The model under review builds one solid part; all positions refer to its coordinate system, in mm. A direction names the side the tool comes from. Give positions to 0.01 mm unless a question says otherwise; leave off trailing zeros. Order: outer loops, then holes, each group sorted by start corner. A loop starts at its lowest first (then second) coordinate and runs counter-clockwise, first axis right, second up. Notation, with made-up numbers: (-12.75, 49) - (21.25, 49) arc R27 ccw to (21.25, 87) - close; hole circle Ø7 at (66, 2). An arc over 180 degrees is marked (long way). Use CSV: the item, a comma, the result in double quotes.
Autodesk Inventor part; units mm, degrees
ref_plane "rail_to_adjusting_block_XY" through (0, 0, -37.5) normal (0, 1, 0) x (1, 0, 0)
ref_plane "rail_to_adjusting_block_YZ" through (0, 0, -37.5) normal (1, 0, 0) x (0, 0, -1)
ref_plane "rail_to_adjusting_block_ZX" through (0, 0, -37.5) normal (0, 0, -1) x (0, 1, 0)
sketch "Sketch_12" plane through (0, 0, 0) normal (0, 0, 1) x (1, 0, 0)
  line L0 (-2.5, 3.7) -> (-2.5, 3.1084)
  line L1 (-2.5, 3.1084) -> (-2.3242, 3.0098)
  arc A0 (-2.1007, 2.75) -> (-2.3242, 3.0098) centre (-2.5686, 2.5736) ccw
  line L2 (-2.1007, 2.75) -> (-1.5, 2.75)
  line L3 (-1.5, 2.75) -> (-1.5, 2.25)
  line L4 (-1.5, 2.25) -> (-2.1007, 2.25)
  arc A1 (-2.3242, 1.9902) -> (-2.1007, 2.25) centre (-2.5686, 2.4264) ccw
  line L5 (-2.3242, 1.9902) -> (-2.5, 1.8917)
  line L6 (-2.5, 1.8917) -> (-2.5, 0.3)
  line L7 (-2.5, 0.3) -> (-2.2, 0)
  line L8 (-2.2, 0) -> (2.2, 0)
  line L9 (2.2, 0) -> (2.5, 0.3)
  line L10 (2.5, 0.3) -> (2.5, 1.8917)
  line L11 (2.5, 1.8917) -> (2.3242, 1.9902)
  arc A2 (2.1007, 2.25) -> (2.3242, 1.9902) centre (2.5686, 2.4263) ccw
  line L12 (2.1007, 2.25) -> (1.5, 2.25)
  line L13 (1.5, 2.25) -> (1.5, 2.75)
  line L14 (1.5, 2.75) -> (2.1007, 2.75)
  arc A3 (2.3242, 3.0098) -> (2.1007, 2.75) centre (2.5686, 2.5737) ccw
  line L15 (2.3242, 3.0098) -> (2.5, 3.1084)
  line L16 (2.5, 3.1084) -> (2.5, 3.7)
  line L17 (2.5, 3.7) -> (2.2, 4)
  line L18 (2.2, 4) -> (-2.2, 4)
  line L19 (-2.2, 4) -> (-2.5, 3.7)
extrude "Extrusion1" add sketch "Sketch_12" along normal mid plane 85
sketch "Sketch2" plane through (-2.2, 4, 42.5) normal (0, 1, 0) x (1, 0, 0)
  point P0 (2.2, 80)
hole "Hole1" at (0, 4, -37.5) direction (0, -1, 0) diameter 2.4 depth 4 counterbore diameter 3.5 counterbore depth 1
pattern_linear "Rectangular Pattern1" count 6 spacing 15 along (0, 0, 1) of "Hole1"
ref_plane "rail_to_adjusting_block_XY" through (0, 0, -37.5) normal (0, 1, 0) x (1, 0, 0)
ref_plane "rail_to_adjusting_block_YZ" through (0, 0, -37.5) normal (1, 0, 0) x (0, 0, -1)
ref_plane "rail_to_adjusting_block_ZX" through (0, 0, -37.5) normal (0, 0, -1) x (0, 1, 0)
ref_plane "screw_1_XY" through (0, 3, 37.5) normal (0, -1, 0) x (1, 0, 0)
ref_plane "screw_1_YZ" through (0, 3, 37.5) normal (1, 0, 0) x (0, 0, 1)
ref_plane "screw_1_ZX" through (0, 3, 37.5) normal (0, 0, 1) x (0, -1, 0)
ref_plane "screw_2_XY" through (0, 3, 22.5) normal (0, -1, 0) x (1, 0, 0)
ref_plane "screw_2_YZ" through (0, 3, 22.5) normal (1, 0, 0) x (0, 0, 1)
ref_plane "screw_2_ZX" through (0, 3, 22.5) normal (0, 0, 1) x (0, -1, 0)
ref_plane "screw_3_XY" through (0, 3, 7.5) normal (0, -1, 0) x (1, 0, 0)
ref_plane "screw_3_YZ" through (0, 3, 7.5) normal (1, 0, 0) x (0, 0, 1)
ref_plane "screw_3_ZX" through (0, 3, 7.5) normal (0, 0, 1) x (0, -1, 0)
ref_plane "screw_4_XY" through (0, 3, -7.5) normal (0, -1, 0) x (1, 0, 0)
ref_plane "screw_4_YZ" through (0, 3, -7.5) normal (1, 0, 0) x (0, 0, 1)
ref_plane "screw_4_ZX" through (0, 3, -7.5) normal (0, 0, 1) x (0, -1, 0)
ref_plane "screw_5_XY" through (0, 3, -22.5) normal (0, -1, 0) x (1, 0, 0)
ref_plane "screw_5_YZ" through (0, 3, -22.5) normal (1, 0, 0) x (0, 0, 1)
ref_plane "screw_5_ZX" through (0, 3, -22.5) normal (0, 0, 1) x (0, -1, 0)
ref_plane "screw_6_XY" through (0, 3, -37.5) normal (0, -1, 0) x (1, 0, 0)
ref_plane "screw_6_YZ" through (0, 3, -37.5) normal (1, 0, 0) x (0, 0, 1)
ref_plane "screw_6_ZX" through (0, 3, -37.5) normal (0, 0, 1) x (0, -1, 0)
ref_plane "to_block_XY" through (0, 4, 21.25) normal (0, 0, 1) x (1, 0, 0)
ref_plane "to_block_YZ" through (0, 4, 21.25) normal (1, 0, 0) x (0, 1, 0)
ref_plane "to_block_ZX" through (0, 4, 21.25) normal (0, 1, 0) x (0, 0, 1)
ref_plane "to_block_2_XY" through (0, 4, -21.25) normal (0, 0, 1) x (1, 0, 0)
ref_plane "to_block_2_YZ" through (0, 4, -21.25) normal (1, 0, 0) x (0, 1, 0)
ref_plane "to_block_2_ZX" through (0, 4, -21.25) normal (0, 1, 0) x (0, 0, 1)
ref_plane "to_kue_XY" through (0, 0, 0) normal (0, 1, 0) x (1, 0, 0)
ref_plane "to_kue_YZ" through (0, 0, 0) normal (1, 0, 0) x (0, 0, -1)
ref_plane "to_kue_ZX" through (0, 0, 0) normal (0, 0, -1) x (0, 1, 0)
properties part number "SSE2B6-85_r"
Item 1: Take a section at B-B, the plane y = 1. Give the boundary of the cut face in (x, z), and give its area (3 significant figures).
Results list:
outline,"(-2.5, -42.5) - (2.5, -42.5) - (2.5, 42.5) - (-2.5, 42.5) - close; hole circle Ø2.4 at (0, -37.5); hole circle Ø2.4 at (0, -22.5); hole circle Ø2.4 at (0, -7.5); hole circle Ø2.4 at (0, 7.5); hole circle Ø2.4 at (0, 22.5); hole circle Ø2.4 at (0, 37.5)"
area,"398 mm2"
Item 2: Clearance check with flat-ended pins moving along their axes: pin 1 (0.6 mm diameter, centred on y = 2.5, z = -2.5, fed in from +X); pin 2 (1.9 mm diameter, centred on x = 0, z = 22.5, fed in from +Y); pin 3 (3 mm diameter, centred on x = 0, z = -22.5, fed in from +Y). State where each tip first meets the part, or that it passes through.
Results list:
pin 1,"stops at x = 2.12"
pin 2,"passes through"
pin 3,"stops at y = 3"
Item 3: Mouldability with a two-part tool opening along Z and no side actions: class faces 3 (the face through (0, 2, -42.5)), 4 (the face through (0, 4, -1)), 5 (the face through (-0.08, 3.49, -24.25)) as pulls with the +Z half, pulls with the -Z half, needs draft (parallel to the pull), parting line crosses it, or undercut.
Results list:
face 3,"pulls with the -Z half"
face 4,"needs draft"
face 5,"undercut"
Item 4: Wall thickness on L1, parallel to Y at x = -1.8, z = -35.5; L2, parallel to X at y = 1.05, z = -7.5; L3, parallel to X at y = 3.5, z = 22.5: over which ranges is each line inside the solid? List them lowest first.
Results list:
L1,"y = 0 to 2.25, 2.75 to 4"
L2,"x = -2.5 to -1.2, 1.2 to 2.5"
L3,"x = -2.5 to -1.75, 1.75 to 2.5"
Item 5: Tool access review of faces 1 (the face through (-0.05, 1.48, -23.7)), 2 (the face through (0, 3, -36)): name each direction out of +Z, -Z, +X, -X, +Y, -Y from which nothing blocks a thin tool from reaching the whole face with its end or side.
Results list:
face 1,"+Y, -Y"
face 2,"+Y"
Item 6: Take a section at C-C, the plane z = -32. Give the boundary of the cut face in (x, y), and give its area (3 significant figures).
Results list:
outline,"(-2.5, 0.3) - (-2.2, 0) - (2.2, 0) - (2.5, 0.3) - (2.5, 1.89) - (2.32, 1.99) arc R0.5 cw to (2.1, 2.25) - (1.5, 2.25) - (1.5, 2.75) - (2.1, 2.75) arc R0.5 cw to (2.32, 3.01) - (2.5, 3.11) - (2.5, 3.7) - (2.2, 4) - (-2.2, 4) - (-2.5, 3.7) - (-2.5, 3.11) - (-2.32, 3.01) arc R0.5 cw to (-2.1, 2.75) - (-1.5, 2.75) - (-1.5, 2.25) - (-2.1, 2.25) arc R0.5 cw to (-2.32, 1.99) - (-2.5, 1.89) - close"
area,"18.5 mm2"
